Source: three-view drawing plus pictorial views. Frame: mm from the lowest corner of the part. Coordinates: 2 decimals unless noted, no trailing zeros. Loops run counter-clockwise (first coordinate to the right, second up) from the corner with the lowest first, then second, coordinate; pieces in that order, holes last. Notation, with made-up numbers: M 78,-16.5 L 130,-16.5 A23 cw 130,7.5 Z; hole C 74,62.25 d9. An arc over 180 degrees is marked long. Use a Markdown table: item, result. Add a question column.
1. Section C-C on y = 2.35. Output: boundary loops of the cut face in (x, z).
2. Section B-B on z = 30.5. Output: boundary loops of the cut face in (x, y).
3. Line query: L1, parallel to X at y = 0.9, z = 30.5; L2, parallel to Z at x = 39.5, y = 2.55; L3, parallel to Z at x = 37.5, y = 2.75. Output: solid intervals per line, ascending. Write a range as [from, to].
4. Section A-A on x = 30.5. Output: boundary loops of the cut face in (y, z), then the cut area to 3 significant figures.
5. Pin query (flat end, axial travel): pin 1 (0.9 mm diameter, centred on y = 1.5, z = 59.5, fed in from -X); pin 2 (0.9 mm diameter, centred on x = 23, y = 1.5, fed in from +Z); pin 3 (1.5 mm diameter, centred on y = 2, z = 35.5, fed in from +X). Return the tip coordinate at first contact, or that it passes through.
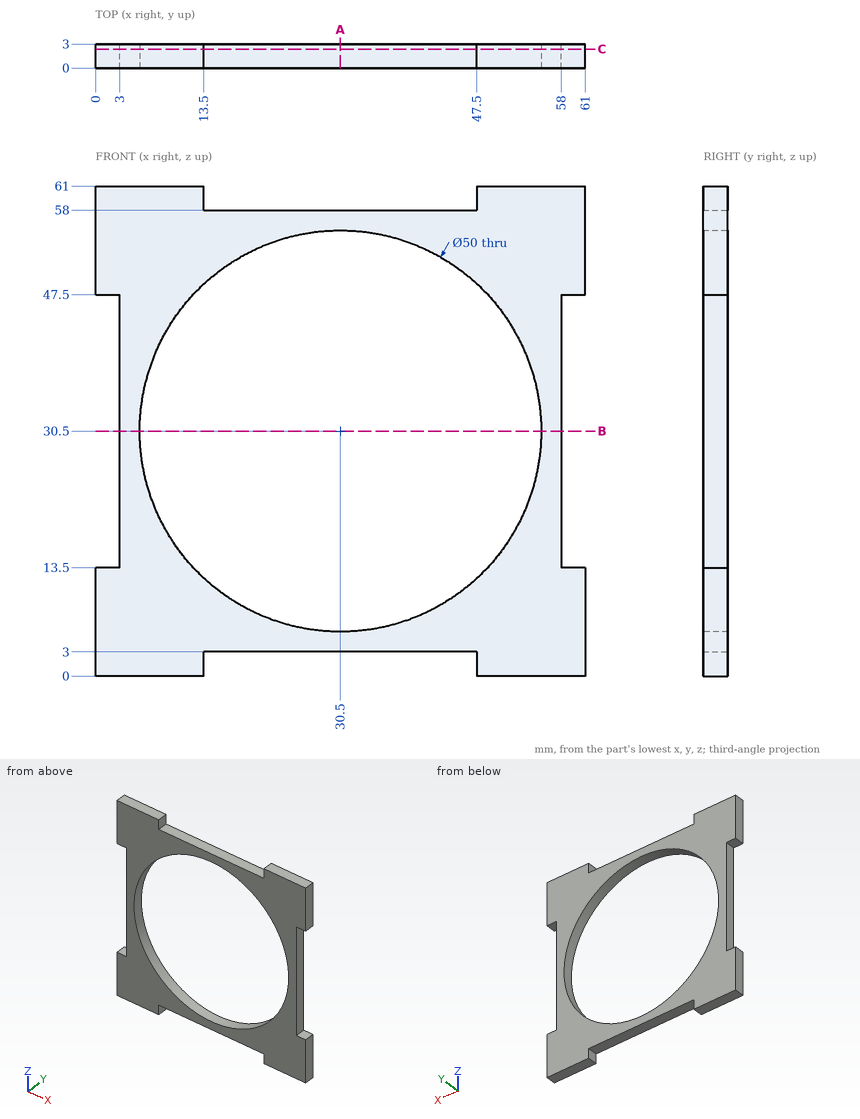
Answers below:
| question | item | result |
|---|---|---|
| 1 | outline | M 0,0 L 13.5,0 L 13.5,3 L 47.5,3 L 47.5,0 L 61,0 L 61,13.5 L 58,13.5 L 58,47.5 L 61,47.5 L 61,61 L 47.5,61 L 47.5,58 L 13.5,58 L 13.5,61 L 0,61 L 0,47.5 L 3,47.5 L 3,13.5 L 0,13.5 Z; hole C 30.5,30.5 d50 |
| 2 | outline | M 3,0 L 5.5,0 L 5.5,3 L 3,3 Z; M 55.5,0 L 58,0 L 58,3 L 55.5,3 Z |
| 3 | L1 | x = [3, 5.5], [55.5, 58] |
| 3 | L2 | z = [3, 7.18], [53.82, 58] |
| 3 | L3 | z = [3, 6.5], [54.5, 58] |
| 4 | outline | M 0,3 L 3,3 L 3,5.5 L 0,5.5 Z; M 0,55.5 L 3,55.5 L 3,58 L 0,58 Z |
| 4 | area | 15.0 mm² |
| 5 | pin 1 | stops at x = 0 |
| 5 | pin 2 | stops at z = 58 |
| 5 | pin 3 | stops at x = 58 |
